Can you work these out from the model? Positions are in its coordinate system, mm. A direction names the side the tool comes from. Give positions to 0.01 mm unless a question says otherwise; leave off trailing zeros. Loops run counter-clockwise (first coordinate to the right, second up) from the corner with the lowest first, then second, coordinate; pieces in that order, holes last.
Autodesk Inventor part; units mm, degrees
ref_plane "Work Plane1" through (-26.704, -73.8176, -12) normal (0, 0, -1) x (0, 1, 0)
ref_plane "YZ Plane" through (0, 0, 0) normal (1, 0, 0) x (0, 1, 0)
ref_plane "XZ Plane" through (0, 0, 0) normal (0, 1, 0) x (-1, 0, 0)
sketch "Sketch1" plane through (0, 0, 0) normal (0, 0, 1) x (1, 0, 0)
  circle A0 centre (-12.704, 28.2207) radius 12
  circle A1 centre (-12.704, -22.5861) radius 12
  line L0 (-12.704, 28.2207) -> (-12.704, -22.5861) construction
  line L1 (4.1406, 2.8173) -> (-27.9996, 2.8173) construction
  line L2 (-24.704, -73.8176) -> (-24.704, 176.1824)
  line L3 (-5.204, -22.5861) -> (-5.204, 28.2207)
  line L4 (-22.204, -2.1827) -> (-6.204, -2.1827)
  line L5 (-6.204, -2.1827) -> (-6.204, 7.8173)
  line L6 (-6.204, 7.8173) -> (-22.204, 7.8173)
  line L7 (-22.204, 7.8173) -> (-22.204, -2.1827)
  circle A2 centre (-9.704, 2.8173) radius 3.5 construction
  circle A3 centre (-19.704, 2.8173) radius 2.5 construction
  point P0 (0, 0)
  point P1 (-12.704, 2.8173)
  dimension "d1" = 10
  dimension "d2" = 5
  dimension "d3" = 7
  dimension "d4" = 5
  dimension "d5" = 10
ref_plane "Work Plane1" through (-26.704, -73.8176, -12) normal (0, 0, -1) x (0, 1, 0)
extrude "Extrusion1" add sketch "Sketch1" against normal up to surface (12 mm away) contours L7 L6 L5 L4
hole "Hole1" at (-9.704, 2.8173, 0) at (-19.704, 2.8173, 0) direction (0, 0, -1) diameter 3.4 end through all
sketch "Sketch2" plane through (-6.204, 7.8173, -12) normal (0, 0, -1) x (-1, 0, 0)
  line L0 (0, -10) -> (0, 0)
  line L1 (16, 0) -> (16, -10)
  line L2 (0, -6.15) -> (16, -6.15)
  line L3 (16, -3.85) -> (0, -3.85)
  line L4 (-10.3445, -5) -> (21.7957, -5) construction
  line L5 (16, -10) -> (0, -10)
  line L6 (0, 0) -> (16, 0)
  point P0 (-6.204, -7.8173)
  dimension "d15" = 2.3
extrude "Extrusion2" add sketch "Sketch2" along normal blind 10 contours L0 L2 L1 L5 | L0 L6 L1 L3
sketch "Sketch3" plane through (-6.204, 7.8173, -22) normal (0, 0, -1) x (-1, 0, 0)
  line L0 (16.25, -3.4123) -> (16.25, -6.5877)
  line L1 (16.25, -6.5877) -> (13.5, -8.1754)
  line L2 (13.5, -8.1754) -> (10.75, -6.5877)
  line L3 (10.75, -6.5877) -> (10.75, -3.4123)
  line L4 (10.75, -3.4123) -> (13.5, -1.8246)
  line L5 (13.5, -1.8246) -> (16.25, -3.4123)
  line L6 (6.25, -3.4123) -> (6.25, -6.5877)
  line L7 (6.25, -6.5877) -> (3.5, -8.1754)
  line L8 (3.5, -8.1754) -> (0.75, -6.5877)
  line L9 (0.75, -6.5877) -> (0.75, -3.4123)
  line L10 (0.75, -3.4123) -> (3.5, -1.8246)
  line L11 (3.5, -1.8246) -> (6.25, -3.4123)
  line L12 (0, -6.15) -> (0, -3.85)
  line L13 (16, -3.85) -> (16, -6.15)
  point P0 (-6.204, -7.8173)
  point P1 (3.5, -5)
  point P2 (13.5, -5)
  point P3 (13.5, -5)
  point P4 (3.5, -5)
  dimension "d18" = 5.5
extrude "Extrusion3" cut sketch "Sketch3" against normal blind 12
sketch "Sketch4" plane through (-22.204, 7.8173, 0) normal (0, 1, 0) x (1, 0, 0)
  line L0 (0, 0) -> (0, 22)
  line L1 (16, 0) -> (0, 0)
  line L2 (16, 0) -> (16, 22)
  line L3 (0, 22) -> (16, 22)
  line L4 (16, 0) -> (16, 22)
  line L5 (16, 19.5) -> (0, 19.5)
  point P0 (22.204, 0)
  point P1 (8, 19.5)
  dimension "d21" = 2.5
hole "Hole2" at (-14.204, 7.8173, -19.5) direction (0, -1, 0) diameter 3.4 end through all
properties part number "belt_holder"
(1) Suppose I cut it at A-A on z = -19.5. Give the number of separate pieces and of enclosed holes in the cut face, plus the area to 3 significant figures.
Returned:
separate pieces: 4
enclosed holes: 0
area: 70.2 mm2
(2) Suppose I cut it at B-B on x = -14.5. List the corners of the cut face in (y, z) for me.
Returned:
outline: (-2.18, -22) - (1.67, -22) - (1.67, -21.17) - (-2.18, -21.17) - close; (-2.18, -17.83) - (1.67, -17.83) - (1.67, -12) - (3.97, -12) - (3.97, -17.83) - (7.82, -17.83) - (7.82, 0) - (-2.18, 0) - close; (3.97, -22) - (7.82, -22) - (7.82, -21.17) - (3.97, -21.17) - close
(3) Thinking about a two-plate mould opening in Y: for faces 4 (the cylindrical face through (-13.55, 5.87, -17.93)), 5 (the flat face through (-14, 7.817, -11)), 6 (the flat face through (-18.348, 0.425, -16.084)), which applies, pulls with the +Y half, pulls with the -Y half, needs draft (parallel to the pull), parting line crosses it, or undercut?
Returned:
face 4: needs draft
face 5: pulls with the +Y half
face 6: undercut
(4) Which directions (+Z, -Z, +X, -X, +Y, -Y) give clear straight access to the entire face, cutting with the end or side of a thin tool? Please do faces 1 (the flat face through (-20.972, 0.374, -16.084)), 2 (the flat face through (-14, 3, 0)), 3 (the flat face through (-15, 1.667, -16)).
Returned:
face 1: -Z
face 2: +Z, +X, -X, +Y, -Y
face 3: -Z, +X, -X
(5) Please list where these lines run through material, in increasing order: probe 1 along X at (y, z) = (2, -11.5); probe 2 along Y at (x, z) = (-16, -16.5); probe 3 along Z at (x, y) = (-18.25, 4.5).
Returned:
probe 1: x = -16.95 to -12.45, -6.95 to -6.2
probe 2: y = -2.18 to 1.67, 3.97 to 7.82
probe 3: z = -10 to 0
(6) Will these pins go through, and if not, where does the flat tip stop? P1, Ø3, axis at x = -15.5, y = 2.5, coming from the -Z side; P2, Ø1.6, axis at y = 2.5, z = -17, coming from the -X side.
Returned:
P1: stops at z = -22
P2: passes through
(7) Suppose I cut it at D-D on z = -11.25. List the corners of the cut face in (x, y) for me (3 decimals).
Returned:
outline: (-22.204, -2.183) - (-6.204, -2.183) - (-6.204, 7.817) - (-22.204, 7.817) - (-22.204, 4.549) - (-19.704, 5.993) - (-16.954, 4.405) - (-16.954, 1.23) - (-19.704, -0.358) - (-22.204, 1.085) - close; hole (-12.454, 1.23) - (-9.704, -0.358) - (-6.954, 1.23) - (-6.954, 4.405) - (-9.704, 5.993) - (-12.454, 4.405) - close
(8) Suppose I cut it at C-C on y = 2.75. List the corners of the cut face in (x, z) for me.
Returned:
outline: (-22.2, -10) - (-21.4, -10) - (-21.4, 0) - (-22.2, 0) - close; (-18.01, -10) - (-16.95, -10) - (-16.95, -12) - (-12.45, -12) - (-12.45, -10) - (-11.4, -10) - (-11.4, 0) - (-18.01, 0) - close; (-8.01, -10) - (-6.95, -10) - (-6.95, -12) - (-6.2, -12) - (-6.2, 0) - (-8.01, 0) - close
